from build123d import *

# Parameters (mm, degrees)
F0_R         = 1.8
F0_R_2       = 13.5
F0_W         = 24.3372796029
F0_H         = 5
F1_DEPTH     = 2
F2_W         = 3
F2_H         = 30
F3_DEPTH     = 27
F4_W         = 20.3372796029
F4_H         = 3
F5_DEPTH     = 25
F7_SIZE      = 25
F8_SIZE      = 14
F9_R         = 4.99999
F10_T1_DEPTH = 2
F10_T3_DEPTH = 32
F6_R         = 6.2
F11_DEPTH    = 25


# Not quite as in the source:
# - a fillet or chamfer that OpenCascade refuses, or shapes differently, is made with other operations: its cross-section is extruded or revolved along the edge and cut away or added
# - a fillet or chamfer is up to 0.001 mm smaller than in the source, because OpenCascade refuses the exact size


with BuildPart() as f1:
    # F0 (on Top) → F1 (new body)
    with BuildSketch(Plane.XY):
        Polygon((21.15, -21.15), (21.15, 21.15), (-21.15, 21.15), (-21.15, 3.85), (-21.15, -21.15), align=None)
        with Locations((-15.5, -15.5)):
            Circle(F0_R, mode=Mode.SUBTRACT)
        with Locations((15.5, -15.5)):
            Circle(F0_R, mode=Mode.SUBTRACT)
        with Locations((-15.5, 15.5)):
            Circle(F0_R, mode=Mode.SUBTRACT)
        Circle(F0_R_2, mode=Mode.SUBTRACT)
        with Locations((15.5, 15.5)):
            Circle(F0_R, mode=Mode.SUBTRACT)
        Polygon((-21.15, -21.15), (-21.15, 3.85), (-45.5, 3.85), (-45.5, -21.15), (-21.1627203971, -21.15), align=None)
        with Locations((-33.3313601986, -23.65)):
            Rectangle(F0_W, F0_H)
    extrude(amount=F1_DEPTH)

    # F2 (on Top) → F3 (join)
    with BuildSketch(Plane.XY):
        with Locations((-23.6627203971, -11.15)):
            Rectangle(F2_W, F2_H)
    extrude(amount=F3_DEPTH)

    # F4 (on face) → F5 (join)
    with BuildSketch(Plane.XY.offset(2)):
        with Locations((-35.3313601986, -24.65)):
            Rectangle(F4_W, F4_H)
    extrude(amount=F5_DEPTH)

    # F7
    f7_edges = [f1.edges().sort_by_distance(p)[0] for p in [
        (-23.66272, 3.85, 27),
    ]]
    chamfer(f7_edges, length=F7_SIZE)

    # F8
    f8_edges = [f1.edges().sort_by_distance(p)[0] for p in [
        (-45.5, 3.85, 1),
    ]]
    chamfer(f8_edges, length=F8_SIZE)

    # F9 (radius 5 in the source; OpenCascade refuses exactly that, so slightly less here)
    f9_edges = [f1.edges().sort_by_distance(p)[0] for p in [
        (-45.5, -10.15, 1),
        (-31.5, 3.85, 1),
        (-21.16272, -26.15, 1),
        (-45.5, -24.65, 27),
    ]]
    fillet(f9_edges, radius=F9_R)

    # F10: fillet of radius 6 on 4 edges, made by hand

    # F10_s2 → F10_t1 (join)
    with BuildSketch(Plane.XY):
        with BuildLine():
            ThreePointArc((-27.15, 3.85), (-22.9073593129, 5.6073593129), (-21.15, 9.85))
            Line((-21.15, 9.85), (-21.15, 3.85))
            Line((-21.15, 3.85), (-27.15, 3.85))
        make_face()
    extrude(amount=F10_T1_DEPTH)

    # F10_s4 → F10_t3 (cut)
    with BuildSketch(Plane.XY.offset(-15)):
        with BuildLine():
            ThreePointArc((21.15, -15.15), (19.3926406871, -19.3926406871), (15.15, -21.15))
            Line((15.15, -21.15), (21.15, -21.15))
            Line((21.15, -21.15), (21.15, -15.15))
        make_face()
        with BuildLine():
            ThreePointArc((15.15, 21.15), (19.3926406871, 19.3926406871), (21.15, 15.15))
            Line((21.15, 15.15), (21.15, 21.15))
            Line((21.15, 21.15), (15.15, 21.15))
        make_face()
        with BuildLine():
            ThreePointArc((-21.15, 15.15), (-19.3926406871, 19.3926406871), (-15.15, 21.15))
            Line((-15.15, 21.15), (-21.15, 21.15))
            Line((-21.15, 21.15), (-21.15, 15.15))
        make_face()
    extrude(amount=F10_T3_DEPTH, mode=Mode.SUBTRACT)

    # F6 (on face) + F5_face1 (on face) → F11 (cut)
    with BuildSketch(Plane(origin=(0, -23.15, 0), x_dir=(-1, 0, 0), z_dir=(0, 1, 0))):
        with Locations((35.5, 13.5)):
            Circle(F6_R)
    with BuildSketch(Plane(origin=(-35.7425668405, -26.15, 13.3714329468), x_dir=(1, 0, 0), z_dir=(0, -1, 0))):
        with BuildLine():
            Line((-9.7574331595, -13.3714329468), (9.5798564434, -13.3714329468))
            Line((9.5798564434, -13.3714329468), (9.5798564434, 13.6285670532))
            Line((9.5798564434, 13.6285670532), (-4.7574431595, 13.6285670532))
            ThreePointArc((-4.7574431595, 13.6285670532), (-8.2929699944, 12.1641038881), (-9.7574331595, 8.6285770532))
            Line((-9.7574331595, 8.6285770532), (-9.7574331595, -13.3714329468))
        make_face()
    extrude(amount=-F11_DEPTH, dir=(0, 1, 0), mode=Mode.SUBTRACT)


solid = f1.part
Geometry: final body of the model. Coordinates: model frame, mm. A direction names the side the tool comes from. Give positions to 0.01 mm unless a question says otherwise; leave off trailing zeros. Order: outer loops, then holes, each group sorted by start corner. A loop starts at its lowest first (then second) coordinate and runs counter-clockwise, first axis right, second up. Notation, with made-up numbers: (-8.75, 34.5) -> (38.25, 34.5) arc R28 cw to (38.25, 69.5) -> close; hole circle Ø8 at (76.25, -13). An arc over 180 degrees is marked (long way). Put each result on its own line as item: value.
Q1. Pin query (flat end, axial travel): pin 1 (24.5 mm diameter, centred on x = 0, y = 0, fed in from -Z); pin 2 (1.5 mm diameter, centred on y = -13, z = 12.5, fed in from -X); pin 3 (5 mm diameter, centred on x = -38.5, y = -20.5, fed in from +Z); pin 4 (2 mm diameter, centred on y = 14, z = 0.5, fed in from -X). Return the tip coordinate at first contact, or that it passes through.
Here are the results:
pin 1: passes through
pin 2: stops at x = -25.16
pin 3: stops at z = 2
pin 4: stops at x = -21.15
Q2. Section D-D, the plane x = -28. Return loops of the section in (y, z).
Here are the results:
outline: (-26.15, 0) -> (3.85, 0) -> (3.85, 2) -> (-23.15, 2) -> (-23.15, 27) -> (-26.15, 27) -> close
Q3. Section C-C, the plane x = 0. Return loops of the section in (y, z).
Here are the results:
outline: (-21.15, 0) -> (-13.5, 0) -> (-13.5, 2) -> (-21.15, 2) -> close; (13.5, 0) -> (21.15, 0) -> (21.15, 2) -> (13.5, 2) -> close
Q4. Section A-A, the plane z = 13.5. Return loops of the section in (x, y).
Here are the results:
outline: (-45.5, -26.15) -> (-41.7, -26.15) -> (-41.7, -23.15) -> (-45.5, -23.15) -> close; (-29.3, -26.15) -> (-26.16, -26.15) arc R5 ccw to (-22.16, -24.15) -> (-22.16, -7.65) -> (-25.16, -7.65) -> (-25.16, -23.15) -> (-29.3, -23.15) -> close
Q5. Draft query along X for faces 4 (the face through (-35, -23.15, 20)), 5 (the face through (-2.93, -13.18, 0.99)), 6 (the face through (-38.42, -3.07, 0.99)). Return one class per face: released by +X, released by -X, zero draft, split by the parting line, or undercut.
Here are the results:
face 4: zero draft
face 5: undercut
face 6: released by -X
Q6. Section B-B, the plane y = 0. Return loops of the section in (x, z), then the cut area to 4 significant figures.
Here are the results:
outline: (-35.35, 0) -> (-13.5, 0) -> (-13.5, 2) -> (-22.16, 2) -> (-22.16, 5.85) -> (-25.16, 5.85) -> (-25.16, 2) -> (-35.35, 2) -> close; (13.5, 0) -> (21.15, 0) -> (21.15, 2) -> (13.5, 2) -> close
area: 70.55 mm^2
Q7. Reachability of faces 1 (the face through (-19, -1, 2)), 2 (the face through (19.346, 19.439, 0.986)), 3 (the face through (-25.163, -13, 12)) from +Z, -Z, +X, -X, +Y, -Y: full face, straight path, thin tool, end or side. Return the list, or none.
Here are the results:
face 1: +Z, +Y
face 2: +Z, -Z, +X, +Y
face 3: +Z, -X, +Y
Q8. Material intervals for L1, parallel to Y at x = -15.5, z = 1.35; L2, parallel to Z at x = -35.5, y = -23.95; L3, parallel to Z at x = 5.5, y = 14, sorted ascending.
Here are the results:
L1: y = -21.15 to -17.3, -13.7 to 13.7, 17.3 to 21.14
L2: z = 0 to 7.3, 19.7 to 27
L3: z = 0 to 2
